Here's the drawing with two shaded views (mm, measured from the low corner). I have some questions. Coordinates: 2 decimals unless noted, no trailing zeros. Write each loop counter-clockwise with the first axis right and the second up, starting at its lowest first coordinate (ties: lowest second). Pieces come first, ordered by that corner, then holes.
Item 1: If we section it at A-A (y = 30): Please give me the cut outline in (x, z).
Item 2: I'm going to push a flat-ended pin straight in: pin 1 Ø9.5 at (x, y) = (140, 90) entering from -Z. Where does the tip first touch, or does it pass through?
Item 3: If I drill on line 1 (X direction, y = 30, z = 12.75); line 2 (Y direction, x = 40, z = 5.5); line 3 (X direction, y = 33, z = 2.75), over which ranges is the centre line in solid material (lowest first)?
Item 4: If we section it at C-C (x = 40): Please give me the cut outline in (y, z).
Item 5: If we section it at B-B (z = 15.5): Please give me the cut outline in (x, y), then the cut area to 3 significant figures.
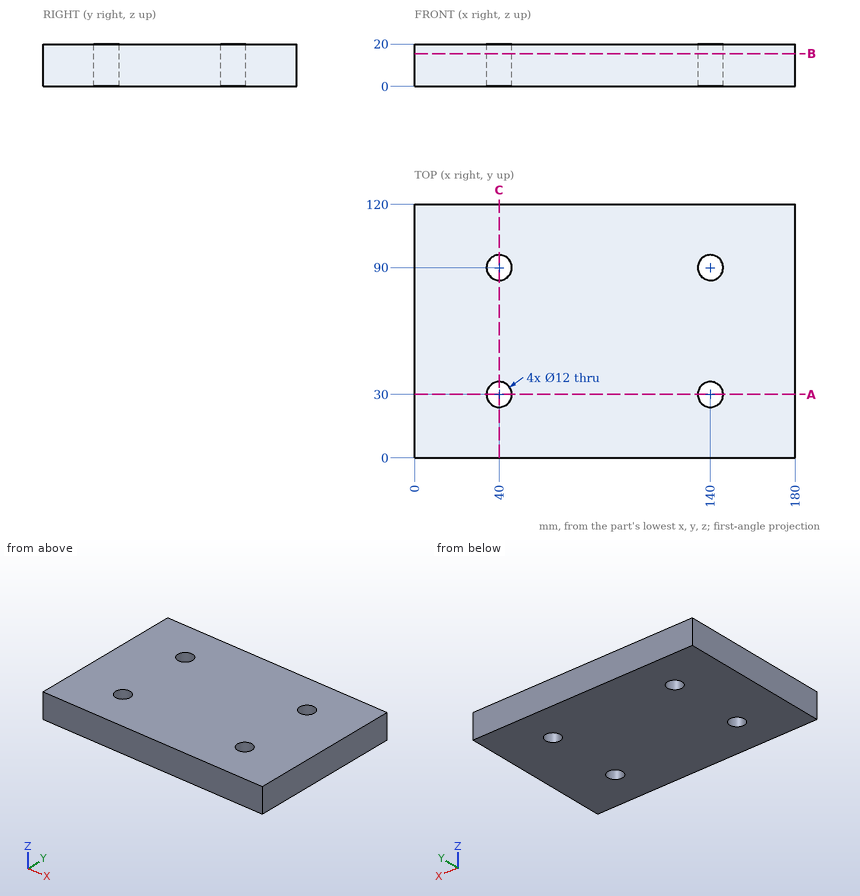
Answer list:
1. outline: (0, 0) - (34, 0) - (34, 20) - (0, 20) - close; (46, 0) - (134, 0) - (134, 20) - (46, 20) - close; (146, 0) - (180, 0) - (180, 20) - (146, 20) - close
2. pin 1: passes through
3. line 1: x = 0 to 34, 46 to 134, 146 to 180
3. line 2: y = 0 to 24, 36 to 84, 96 to 120
3. line 3: x = 0 to 34.8, 45.2 to 134.8, 145.2 to 180
4. outline: (0, 0) - (24, 0) - (24, 20) - (0, 20) - close; (36, 0) - (84, 0) - (84, 20) - (36, 20) - close; (96, 0) - (120, 0) - (120, 20) - (96, 20) - close
5. outline: (0, 0) - (180, 0) - (180, 120) - (0, 120) - close; hole circle Ø12 at (40, 30); hole circle Ø12 at (40, 90); hole circle Ø12 at (140, 30); hole circle Ø12 at (140, 90)
5. area: 21,100 mm2
